Check sheet for the modelled part. Datum: model origin and axes. Units: mm. A direction names the side the tool comes from. Round coordinates to 2 decimals unless told otherwise and drop trailing zeros. Write each loop counter-clockwise with the first axis right and the second up, starting at its lowest first coordinate (ties: lowest second). Pieces come first, ordered by that corner, then holes. Notation, with made-up numbers: (16.5, 6.5) - (38.5, 6.5) arc R31 ccw to (38.5, 40.5) - close; hole circle Ø5 at (-37, 76). An arc over 180 degrees is marked (long way). Answer as a JSON object with one key per item and string values. Group by question number.
Item 1: Set-up check for faces 5 (the flat face through (1, -6, 0)), 6 (the flat face through (2, 5, -4)): record each of +Z, -Z, +X, -X, +Y, -Y from which the full face is reachable in a straight line by a thin tool's end or side.
Item 2: Thickness scan on line 1 (Y direction, x = 0.7, z = 11.11); line 2 (Z direction, x = 0.95, y = 0.75); line 3 (Z direction, x = 1.75, y = 1.75). Record the ranges inside material, lowest first.
Item 3: Gauge pin test, flat end, axial feed: P1, Ø3, axis at y = 1, z = 11.11, coming from the -X side. Record the tip position at first contact, or that the pin passes through.
Item 4: Sectioned sample at B-B on z = -11.11. Record the boundary of the cut face in (x, y), plus the area to 3 significant figures.
Item 5: Sectioned sample at D-D on z = 11.5. Record the boundary of the cut face in (x, y), plus the area to 3 significant figures.
Item 6: Sectioned sample at A-A on y = 1. Record the boundary of the cut face in (x, z), plus the area to 3 significant figures.
Item 7: Sectioned sample at C-C on x = 0.8. Record the boundary of the cut face in (y, z), plus the area to 3 significant figures.
Item 8: Release check for a two-part mould opening along Z. For faces 1 (the flat face through (1, 0, 20)), 2 (the flat face through (2, 5, 4)), 3 (the cylindrical face through (1.521, 0.521, 9.955)), 4 (the flat face through (1, 6, -12)) record: pulls with the +Z half, pulls with the -Z half, needs draft (parallel to the pull), parting line crosses it, or undercut.
```python
from build123d import *

# Parameters (mm, degrees)
SKETCH1_W           = 40
SKETCH1_H           = 12
BOSS_EXTRUDE1_DEPTH = 3
SKETCH2_R           = 1.25
SKETCH2_W           = 8
SKETCH2_H           = 2
CUT_EXTRUDE1_DEPTH  = 5


with BuildPart() as part:
    # Sketch1 → Boss-Extrude1 (new body)
    with BuildSketch(Plane(origin=(0, 0, 0), x_dir=(0, 0, -1), z_dir=(1, 0, 0))):
        Rectangle(SKETCH1_W, SKETCH1_H)
    extrude(amount=BOSS_EXTRUDE1_DEPTH)

    # Sketch2 → Cut-Extrude1 (cut)
    with BuildSketch(Plane(origin=(3, 0, 0), x_dir=(0, 0, -1), z_dir=(1, 0, 0))):
        with Locations((-11.11, 1)):
            Circle(SKETCH2_R)
        with Locations((0, 5)):
            Rectangle(SKETCH2_W, SKETCH2_H)
    cut_extrude1 = extrude(amount=-CUT_EXTRUDE1_DEPTH, mode=Mode.SUBTRACT)

    # Mirror1: Cut-Extrude1 across plane
    add(cut_extrude1.mirror(Plane.XY), mode=Mode.SUBTRACT)


solid = part.part
```
Completed:
{
 "1": {"face 5": "+Z, -Z, +X, -X, -Y", "face 6": "+X, -X, +Y"},
 "2": {"line 1": "-6 to -0.25, 2.25 to 6", "line 2": "-20 to -12.33, -9.89 to 9.89, 12.33 to 20", "line 3": "-20 to -12.11, -10.11 to 10.11, 12.11 to 20"},
 "3": {"P1": "x = 0"},
 "4": {"outline": "(0, -6) - (3, -6) - (3, -0.25) - (0, -0.25) - close; (0, 2.25) - (3, 2.25) - (3, 6) - (0, 6) - close", "area": "28.5 mm²"},
 "5": {"outline": "(0, -6) - (3, -6) - (3, -0.19) - (0, -0.19) - close; (0, 2.19) - (3, 2.19) - (3, 6) - (0, 6) - close", "area": "28.9 mm²"},
 "6": {"outline": "(0, -20) - (3, -20) - (3, -12.36) - (0, -12.36) - close; (0, -9.86) - (3, -9.86) - (3, 9.86) - (0, 9.86) - close; (0, 12.36) - (3, 12.36) - (3, 20) - (0, 20) - close", "area": "105 mm²"},
 "7": {"outline": "(-6, -20) - (6, -20) - (6, -4) - (4, -4) - (4, 4) - (6, 4) - (6, 20) - (-6, 20) - close; hole circle Ø2.5 at (1, -11.11); hole circle Ø2.5 at (1, 11.11)", "area": "454 mm²"},
 "8": {"face 1": "pulls with the +Z half", "face 2": "undercut", "face 3": "undercut", "face 4": "needs draft"}
}
